from build123d import *

# Parameters (mm, degrees)
F1_DEPTH  = 15
F2_W      = 12
F2_H      = 10
F3_DEPTH  = 9
F4_R      = 0.8
F5_DEPTH  = 1
F6_R      = 1.5
F7_DEPTH  = 3.8
F8_R      = 2.5
F9_DEPTH  = 1.3
F10_W     = 0.3
F10_H     = 1.5
F11_DEPTH = 1.9


with BuildPart() as f1:
    # F0 (on Top) → F1 (new body)
    with BuildSketch(Plane.XY):
        with BuildLine():
            Line((3.316625, 5), (-3.316625, 5))
            ThreePointArc((-3.316625, 5), (-6, 0), (-3.316625, -5))
            Line((-3.316625, -5), (3.316625, -5))
            ThreePointArc((3.316625, -5), (6, 0), (3.316625, 5))
        make_face()
    extrude(amount=F1_DEPTH)

    # F2 (on face) → F3 (join)
    with BuildSketch(Plane(origin=(0, 0, 0), x_dir=(1, 0, 0), z_dir=(0, 0, -1))):
        Rectangle(F2_W, F2_H)
    extrude(amount=F3_DEPTH)

    # F4 (on face) → F5 (cut)
    with BuildSketch(Plane(origin=(0, 0, -9), x_dir=(1, 0, 0), z_dir=(0, 0, -1))):
        with Locations((-4.5, 0)):
            Circle(F4_R)
        with Locations((4.5, 0)):
            Circle(F4_R)
    extrude(amount=-F5_DEPTH, mode=Mode.SUBTRACT)

    # F6 (on face) → F7 (join)
    with BuildSketch(Plane(origin=(0, 0, -9), x_dir=(1, 0, 0), z_dir=(0, 0, -1))):
        Circle(F6_R)
    extrude(amount=F7_DEPTH)

    # F8 (on face) → F9 (join)
    with BuildSketch(Plane.XY.offset(15)):
        Circle(F8_R)
    extrude(amount=F9_DEPTH)

    # F10 (on face) → F11 (join)
    with BuildSketch(Plane.XY.offset(15)):
        with Locations((3.95, 0)):
            Rectangle(F10_W, F10_H)
        with Locations((-3.95, 0)):
            Rectangle(F10_W, F10_H)
    extrude(amount=F11_DEPTH)


solid = f1.part
Geometry check sheet. Reference: the model listing, model coordinates, mm. A direction names the side the tool comes from. Round coordinates to 2 decimals unless told otherwise and drop trailing zeros. Write each loop counter-clockwise with the first axis right and the second up, starting at its lowest first coordinate (ties: lowest second). Pieces come first, ordered by that corner, then holes.
Item 1: Section check D-D (x = -4.5). Record the boundary of the cut face in (y, z).
Determined:
outline: (-5, -9) - (-0.8, -9) - (-0.8, -8) - (0.8, -8) - (0.8, -9) - (5, -9) - (5, 0) - (3.97, 0) - (3.97, 15) - (-3.97, 15) - (-3.97, 0) - (-5, 0) - close
Item 2: Material ranges on line 1 along X through (y, z) = (0, -8.8); line 2 along Y through (x, z) = (-4.5, -8.55); line 3 along Z through (x, y) = (-1, -1), recorded low to high.
Determined:
line 1: x = -6 to -5.3, -3.7 to 3.7, 5.3 to 6
line 2: y = -5 to -0.8, 0.8 to 5
line 3: z = -12.8 to 16.3
Item 3: Access from +Z, -Z, +X, -X, +Y, -Y to the whole of each face (thin tool, end or side, straight path). Record for faces 4 (the face through (-6, 0, 7)), 5 (the face through (4, 0, -8)), 6 (the face through (-5, 4, 0)), 7 (the face through (-3.8, 0, 16)), 8 (the face through (5, -4, 0)).
Determined:
face 4: +Z, -X
face 5: -Z
face 6: +Z, -X, +Y
face 7: +Z, +Y, -Y
face 8: +Z, +X, -Y
Item 4: Mould release check, pull along Y, two halves, no side actions. Record for faces 1 (the face through (3.7, 0, -8.5)), 2 (the face through (6, 0, 7)), 3 (the face through (3, 0, 15)): +Y half, -Y half, draft (parallel to the pull), parting line (faces both ways), or undercut.
Determined:
face 1: undercut
face 2: parting line
face 3: draft
Item 5: Section check A-A (x = 0). Record the boundary of the cut face in (y, z).
Determined:
outline: (-5, -9) - (-1.5, -9) - (-1.5, -12.8) - (1.5, -12.8) - (1.5, -9) - (5, -9) - (5, 15) - (2.5, 15) - (2.5, 16.3) - (-2.5, 16.3) - (-2.5, 15) - (-5, 15) - close
Item 6: Go/stop test with flat-tipped pins: pin 1 Ø2 at (x, y) = (4.5, 0) entering from -Z; pin 2 Ø0.8 at (y, z) = (-0.5, 15.5) entering from -X; pin 3 Ø1.3 at (x, y) = (-5, 3) entering from +Z. Record where each tip stops, or that it passes through.
Determined:
pin 1: stops at z = -9
pin 2: stops at x = -4.1
pin 3: stops at z = 15
Item 7: Section check B-B (z = 7.5). Record the boundary of the cut face in (x, y).
Determined:
outline: (-3.32, -5) - (3.32, -5) arc R6 ccw to (3.32, 5) - (-3.32, 5) arc R6 ccw to start
Item 8: Section check C-C (y = 3.25). Record the boundary of the cut face in (x, z).
Determined:
outline: (-6, -9) - (6, -9) - (6, 0) - (5.04, 0) - (5.04, 15) - (-5.04, 15) - (-5.04, 0) - (-6, 0) - close
